Geometry check sheet. Reference: the model listing, model coordinates, mm. A direction names the side the tool comes from. Coordinates: 2 decimals unless noted, no trailing zeros. Write each loop counter-clockwise with the first axis right and the second up, starting at its lowest first coordinate (ties: lowest second). Pieces come first, ordered by that corner, then holes.
from build123d import *

# Parameters (mm, degrees)
SKETCH1_R           = 1.5
BOSS_EXTRUDE1_DEPTH = 5
FILLET1_R           = 2
SKETCH2_W           = 7.277082667
SKETCH2_H           = 36
CUT_EXTRUDE1_DEPTH  = 10


with BuildPart() as part:
    # Sketch1 → Boss-Extrude1 (new body)
    with BuildSketch(Plane(origin=(0, 0, 0), x_dir=(1, 0, 0), z_dir=(0, 1, 0))):
        Polygon((0, 31), (0, 36), (29, 36), (29, 0), (0, 0), (0, 5), (25, 5), (25, 31), align=None)
        with Locations((26, 2.5)):
            Circle(SKETCH1_R, mode=Mode.SUBTRACT)
        with Locations((26, 33.5)):
            Circle(SKETCH1_R, mode=Mode.SUBTRACT)
        with Locations((3, 33.5)):
            Circle(SKETCH1_R, mode=Mode.SUBTRACT)
        with Locations((3, 2.5)):
            Circle(SKETCH1_R, mode=Mode.SUBTRACT)
    extrude(amount=BOSS_EXTRUDE1_DEPTH)

    # Fillet1
    fillet1_edges = [part.edges().sort_by_distance(p)[0] for p in [
        (0, 2.5, -36),
        (29, 2.5, -36),
        (29, 2.5, 0),
        (0, 2.5, 0),
        (0, 2.5, -5),
        (25, 2.5, -5),
        (25, 2.5, -31),
        (0, 2.5, -31),
    ]]
    fillet(fillet1_edges, radius=FILLET1_R)

    # Sketch2 → Cut-Extrude1 (cut)
    with BuildSketch(Plane(origin=(0, 5, 0), x_dir=(1, 0, 0), z_dir=(0, 1, 0))):
        with Locations((2.323033499, 18)):
            Rectangle(SKETCH2_W, SKETCH2_H)
    extrude(amount=-CUT_EXTRUDE1_DEPTH, mode=Mode.SUBTRACT)


solid = part.part
1. Sectioned sample at A-A, the plane z = -33.5. Record the boundary of the cut face in (x, y).
Computed values:
outline: (5.96, 0) - (24.5, 0) - (24.5, 5) - (5.96, 5) - close; (27.5, 0) - (29, 0) - (29, 5) - (27.5, 5) - close
2. Gauge pin test, flat end, axial feed: pin 1 Ø1.5 at (y, z) = (2.5, -21.5) entering from -X. Record the tip position at first contact, or that the pin passes through.
Computed values:
pin 1: stops at x = 25
3. Access from +Z, -Z, +X, -X, +Y, -Y to the whole of each face (thin tool, end or side, straight path). Record for faces 1 (the cylindrical face through (28.4, 2.54, -35.43)), 2 (the flat face through (15, 2, -31)).
Computed values:
face 1: -Z, +X, +Y, -Y
face 2: -X, +Y, -Y
4. Sectioned sample at B-B, the plane x = 26. Record the boundary of the cut face in (y, z), and give its area (3 significant figures).
Computed values:
outline: (0, -36) - (5, -36) - (5, -35) - (0, -35) - close; (0, -32) - (5, -32) - (5, -4) - (0, -4) - close; (0, -1) - (5, -1) - (5, 0) - (0, 0) - close
area: 150 mm2
5. Sectioned sample at D-D, the plane y = 3.3. Record the boundary of the cut face in (x, z).
Computed values:
outline: (5.96, -36) - (27, -36) arc R2 ccw to (29, -34) - (29, -2) arc R2 ccw to (27, 0) - (5.96, 0) - (5.96, -5) - (23, -5) arc R2 cw to (25, -7) - (25, -29) arc R2 cw to (23, -31) - (5.96, -31) - close; hole circle Ø3 at (26, -33.5); hole circle Ø3 at (26, -2.5)
6. Sectioned sample at C-C, the plane x = 18.75. Record the boundary of the cut face in (y, z).
Computed values:
outline: (0, -36) - (5, -36) - (5, -31) - (0, -31) - close; (0, -5) - (5, -5) - (5, 0) - (0, 0) - close
7. Draft check along Z on faces 3 (the flat face through (17, 2, 0)), 4 (the cylindrical face through (24.43, 2.54, -5.6)), 5 (the flat face through (25.3, 5, -18.3)), 6 (the flat face through (16, 2, -36)). Enter one of: released by +Z, released by -Z, zero draft, split by the parting line, or undercut.
Computed values:
face 3: released by +Z
face 4: undercut
face 5: zero draft
face 6: released by -Z
8. Thickness scan on line 1 along Z through (x, y) = (26, 2.3); line 2 along X through (y, z) = (1.1, -33.5); line 3 along Z through (x, y) = (9, 3.65). Record the ranges inside material, lowest first.
Computed values:
line 1: z = -36 to -35, -32 to -4, -1 to 0
line 2: x = 5.96 to 24.5, 27.5 to 29
line 3: z = -36 to -31, -5 to 0
